CAD build for the part. Positions are in the model's coordinates, mm. A direction names the side the tool comes from. Coordinates: 2 decimals unless noted, no trailing zeros. Write each loop counter-clockwise with the first axis right and the second up, starting at its lowest first coordinate (ties: lowest second). Pieces come first, ordered by that corner, then holes.
```python
from build123d import *

# Parameters (mm, degrees)
F0_W        = 50
F0_H        = 75
F1_DEPTH    = 50
F2_W        = 44
F2_H        = 69
F3_DEPTH    = 47
F4_T1_DEPTH = 311.5948348929
F5_R        = 4
F5_R_2      = 2
F6_DEPTH    = 3
F7_R        = 6.5
F8_DEPTH    = 3


# Not quite as in the source:
# - a fillet or chamfer that OpenCascade refuses, or shapes differently, is made with other operations: its cross-section is extruded or revolved along the edge and cut away or added


with BuildPart() as f1:
    # F0 (on Front) → F1 (new body)
    with BuildSketch(Plane.XZ):
        Rectangle(F0_W, F0_H)
    extrude(amount=F1_DEPTH)

    # F2 (on face) → F3 (cut)
    with BuildSketch(Plane.XZ.offset(50)):
        Rectangle(F2_W, F2_H)
    extrude(amount=-F3_DEPTH, mode=Mode.SUBTRACT)

    # F4: chamfer of 46 on 1 edges, made by hand

    # F4_s2 → F4_t1 (cut)
    with BuildSketch(Plane.XY.offset(-155.7974174464)):
        Polygon((-25, -4), (21, -50), (-25, -50), align=None)
    extrude(amount=F4_T1_DEPTH, mode=Mode.SUBTRACT)

    # F5 (on face) → F6 (cut, through all)
    with BuildSketch(Plane.XZ.offset(3)):
        with Locations((-15.5, 22.5)):
            Circle(F5_R)
        with Locations((15.5, 22.5)):
            Circle(F5_R)
        with Locations((15.5, -22.5)):
            Circle(F5_R)
        with Locations((-15.5, -22.5)):
            Circle(F5_R)
        Circle(F5_R_2)
    extrude(amount=-F6_DEPTH, mode=Mode.SUBTRACT)

    # F7 (on face) → F8 (cut, through all)
    with BuildSketch(Plane.YZ.offset(25)):
        with Locations((-25, 0)):
            Circle(F7_R)
    extrude(amount=-F8_DEPTH, mode=Mode.SUBTRACT)


solid = f1.part
```
Item 1: Two-plate mould, pull along Z, no slides. Class faces 3 (the cylindrical face through (12.55, -1.52, 25.2)), 4 (the flat face through (-23, -6, 0)), 5 (the flat face through (5, -19, 37.5)): +Z half, -Z half, draft (parallel to the pull), parting line (faces both ways), or undercut.
Item 2: Which spindle directions (+Z, -Z, +X, -X, +Y, -Y) get a long thin tool onto all of the face, cutting with end or side? Do faces 1 (the flat face through (23, -50, 1)), 2 (the flat face through (-5, -3, 0)). Say none if no direction does.
Item 3: Saw through at B-B, the plane x = -15.5. Write the cut outline in (y, z), and give its area (3 significant figures).
Item 4: Saw through at A-A, the plane z = 0. Write the cut outline in (x, y), and give its area (4 significant figures).
Item 5: Saw through at D-D, the plane x = 0. Write the cut outline in (y, z).
Item 6: Saw through at C-C, the plane y = -27. Write the cut outline in (x, z), and give its area (3 significant figures).
Item 7: Wall check: line 1 along Z through (x, y) = (15.5, -1); line 2 along Z through (x, y) = (7.5, -33); line 3 along X through (y, z) = (-1, -22). Give the ranges that are in metal, low to high.
Item 8: Flat gauge pins, fed straight in: pin 1 Ø4 at (y, z) = (-28.5, -26) entering from -X; pin 2 Ø23.5 at (y, z) = (-18.5, -1.5) entering from -X; pin 3 Ø10 at (x, z) = (-10, 15) entering from -Y. Where does each tip first touch, or does it go through?
Working result:
1. face 3: undercut
1. face 4: draft
1. face 5: +Z half
2. face 1: +Z, -Z, +X, -X, -Y
2. face 2: -Y
3. outline: (-13.5, -37.5) - (0, -37.5) - (0, -26.5) - (-3, -26.5) - (-3, -34.5) - (-13.5, -34.5) - close; (-13.5, 34.5) - (-3, 34.5) - (-3, 26.5) - (0, 26.5) - (0, 37.5) - (-13.5, 37.5) - close; (-3, -18.5) - (0, -18.5) - (0, 18.5) - (-3, 18.5) - close
3. area: 240 mm2
4. outline: (-25, -4) - (-22, -7) - (-22, -3) - (-2, -3) - (-2, 0) - (-25, 0) - close; (2, -3) - (22, -3) - (22, -18.5) - (25, -18.5) - (25, 0) - (2, 0) - close; (22, -50) - (25, -50) - (25, -31.5) - (22, -31.5) - close
4. area: 247.5 mm2
5. outline: (-29, -37.5) - (0, -37.5) - (0, -2) - (-3, -2) - (-3, -34.5) - (-29, -34.5) - close; (-29, 34.5) - (-3, 34.5) - (-3, 2) - (0, 2) - (0, 37.5) - (-29, 37.5) - close
6. outline: (-2, -37.5) - (25, -37.5) - (25, -6.18) - (22, -6.18) - (22, -34.5) - (-2, -34.5) - close; (-2, 34.5) - (22, 34.5) - (22, 6.18) - (25, 6.18) - (25, 37.5) - (-2, 37.5) - close
6. area: 332 mm2
7. line 1: z = -37.5 to -26.5, -18.5 to 18.5, 26.5 to 37.5
7. line 2: z = -37.5 to -34.5, 34.5 to 37.5
7. line 3: x = -25 to -19.47, -11.53 to 11.53, 19.47 to 25
8. pin 1: stops at x = 22
8. pin 2: stops at x = -22.25
8. pin 3: stops at y = -3
